from build123d import *

# Parameters (mm, degrees)
F0_W     = 100
F0_H     = 70
F1_DEPTH = 12
F2_R     = 19.3
F2_R_2   = 1.5
F3_DEPTH = 12.001
F5_D     = 8


with BuildPart() as f1:
    # F0 (on Front) → F1 (new body)
    with BuildSketch(Plane.XZ):
        Rectangle(F0_W, F0_H)
    extrude(amount=F1_DEPTH)

    # F2 (on face) → F3 (cut, through all)
    with BuildSketch(Plane.XZ.offset(12)):
        Circle(F2_R)
        with Locations((-23.622, 23.622)):
            Circle(F2_R_2)
        with Locations((23.622, 23.622)):
            Circle(F2_R_2)
        with Locations((23.622, -23.622)):
            Circle(F2_R_2)
        with Locations((-23.622, -23.622)):
            Circle(F2_R_2)
    extrude(amount=-F3_DEPTH, mode=Mode.SUBTRACT)

    # F5 (through all)
    with Locations(Plane.XY.offset(35)):
        with Locations((-40, -6), (40, -6)):
            Hole(F5_D / 2)


solid = f1.part
The model under review builds one solid part; all positions refer to its coordinate system, in mm. Coordinates: 2 decimals unless noted, no trailing zeros. Write each loop counter-clockwise with the first axis right and the second up, starting at its lowest first coordinate (ties: lowest second). Pieces come first, ordered by that corner, then holes. Notation, with made-up numbers: (87.5, 54.5) -> (117.5, 54.5) arc R34 cw to (117.5, 87.5) -> close; hole circle Ø1 at (40, 21.5). An arc over 180 degrees is marked (long way). Answer in a Markdown table with one row per item.
1. Wall thickness on probe 1 along X at (y, z) = (-4.75, -23.5); probe 2 along X at (y, z) = (-8.25, 21); probe 3 along X at (y, z) = (-5.25, 27): over which ranges is each line inside the solid? List them lowest first. Write a range as [from, to].
Answers below:
| item | result |
|---|---|
| probe 1 | x = [-50, -43.8], [-36.2, -25.12], [-22.13, 22.13], [25.12, 36.2], [43.8, 50] |
| probe 2 | x = [-50, -43.31], [-36.69, 36.69], [43.31, 50] |
| probe 3 | x = [-50, -43.93], [-36.07, 36.07], [43.93, 50] |
2. We need section B-B, the plane y = -3.75. State the section outline as (x, z) points, and give its area (3 significant figures).
Answers below:
| item | result |
|---|---|
| outline | (-50, -35) -> (-43.31, -35) -> (-43.31, 35) -> (-50, 35) -> close; (-36.69, -35) -> (36.69, -35) -> (36.69, 35) -> (-36.69, 35) -> close; (43.31, -35) -> (50, -35) -> (50, 35) -> (43.31, 35) -> close; hole circle Ø3 at (-23.62, -23.62); hole circle Ø3 at (-23.62, 23.62); hole circle Ø38.6 at (0, 0); hole circle Ø3 at (23.62, -23.62); hole circle Ø3 at (23.62, 23.62) |
| area | 4,880 mm^2 |
3. Clearance check with a flat-ended pin moving along its axis: pin 1 Ø6.5 at (x, y) = (40, -6) entering from -Z. State where the tip first meets the part, or that it passes through.
Answers below:
| item | result |
|---|---|
| pin 1 | passes through |
4. We need section C-C, the plane x = 0. State the section outline as (y, z) points, and give its area (3 significant figures).
Answers below:
| item | result |
|---|---|
| outline | (-12, -35) -> (0, -35) -> (0, -19.3) -> (-12, -19.3) -> close; (-12, 19.3) -> (0, 19.3) -> (0, 35) -> (-12, 35) -> close |
| area | 377 mm^2 |
5. We need section A-A, the plane z = 0. State the section outline as (x, y) points, and give its area (3 significant figures).
Answers below:
| item | result |
|---|---|
| outline | (-50, -12) -> (-19.3, -12) -> (-19.3, 0) -> (-50, 0) -> close; (19.3, -12) -> (50, -12) -> (50, 0) -> (19.3, 0) -> close; hole circle Ø8 at (-40, -6); hole circle Ø8 at (40, -6) |
| area | 636 mm^2 |
6. Draft analysis for pull direction Z (two halves, no side actions). For faces 1 (the cylindrical face through (23.427, -6.084, -22.135)), 2 (the flat face through (-50, -6, 0)), 3 (the cylindrical face through (23.297, -6.084, 22.158)), 4 (the flat face through (-1, -6, 35)), state which applies: +Z half, -Z half, draft (parallel to the pull), parting line (faces both ways), or undercut.
Answers below:
| item | result |
|---|---|
| face 1 | undercut |
| face 2 | draft |
| face 3 | undercut |
| face 4 | +Z half |
7. We need section D-D, the plane z = -8.5. State the section outline as (x, y) points.
Answers below:
| item | result |
|---|---|
| outline | (-50, -12) -> (-17.33, -12) -> (-17.33, 0) -> (-50, 0) -> close; (17.33, -12) -> (50, -12) -> (50, 0) -> (17.33, 0) -> close; hole circle Ø8 at (-40, -6); hole circle Ø8 at (40, -6) |
